Geometry check sheet. Reference: drawing and pictorial views, mm from the part's lowest x, y, z. A direction names the side the tool comes from. Give positions to 0.01 mm unless a question says otherwise; leave off trailing zeros. Order: outer loops, then holes, each group sorted by start corner. A loop starts at its lowest first (then second) coordinate and runs counter-clockwise, first axis right, second up.
Item 1: Material ranges on line 1 along Y through (x, z) = (15.5, 2) (1 decimal); line 2 along Y through (x, z) = (20.5, 8.5) (1 decimal); line 3 along Z through (x, y) = (21, 14), recorded low to high.
Item 2: Sectioned sample at C-C on x = 5. Record the boundary of the cut face in (y, z).
Item 3: Access from +Z, -Z, +X, -X, +Y, -Y to the whole of each face (thin tool, end or side, straight path). Record for the marked faces 1 and 2.
Item 4: Gauge pin test, flat ends, axial feed: P1, Ø10, axis at x = 15.88, y = 6.4, coming from the +Z side; P2, Ø5, axis at x = 13.5, z = 8, coming from the -Y side; P3, Ø5, axis at x = 8, z = 7, coming from the +Y side; P4, Ø1.5, axis at y = 14.5, z = 8, coming from the +X side. Record the tip position at first contact, or that the pin passes through.
Item 5: Sectioned sample at A-A on x = 16.5. Count the separate pieces of the cut face and the enclosed holes in it, and give its area (3 significant figures).
Item 6: Release check for a two-part mould opening along X. For the marked faces 3, 4 and 5 record: released by +X, released by -X, zero draft, split by the parting line, or undercut.
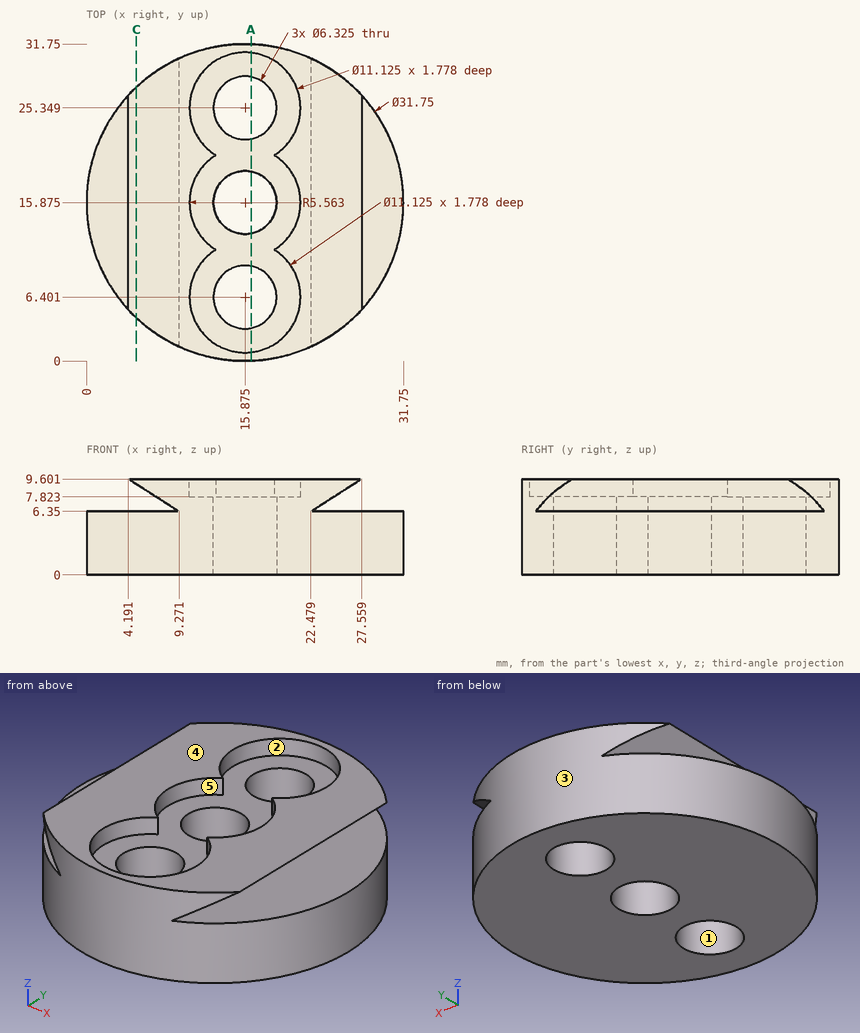
Report:
1. line 1: y = 0 to 3.3, 9.5 to 12.7, 19 to 22.2, 28.5 to 31.7
1. line 2: y = 0.7 to 3.3, 9.5 to 12.8, 19 to 22.3, 28.4 to 31.1
1. line 3: z = 0 to 7.82
2. outline: (4.31, 0) - (27.44, 0) - (27.44, 6.35) - (4.31, 6.35) - close; (4.31, 9.08) - (27.44, 9.08) - (27.44, 9.6) - (4.31, 9.6) - close
3. face 1: +Z, -Z
3. face 2: +Z
4. P1: stops at z = 7.82
4. P2: stops at y = 0
4. P3: stops at y = 30.81
4. P4: stops at x = 26.23
5. separate pieces: 4
5. enclosed holes: 0
5. area: 106 mm2
6. face 3: split by the parting line
6. face 4: zero draft
6. face 5: undercut
